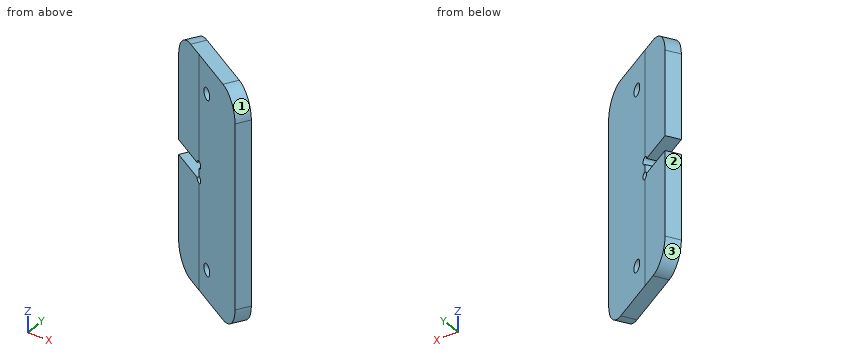
```python
from build123d import *

# Parameters (mm, degrees)
BOSS_EXTRUDE1_DEPTH      = 44.5
BOSS_EXTRUDE1_DEPTH_BACK = 50.5
SKETCH2_W                = 16.785504055
SKETCH2_H                = 44.5
BOSS_EXTRUDE2_DEPTH      = 6
FILLET1_R                = 10
SKETCH3_R                = 1.5
SKETCH3_R_2              = 2.4
CUT_EXTRUDE1_DEPTH       = 549.376643642


with BuildPart() as part:
    # Sketch1 → Boss-Extrude1 (new, two sides: drawn at the far end of the back side and taken through both)
    with BuildSketch(Plane.XY.offset(-25).offset(-BOSS_EXTRUDE1_DEPTH_BACK)):
        Polygon((724, 137.920851515), (698.573213095, 153.84185989), (701.75741477, 158.927217271), (727.184201675, 143.006208896), align=None)
    extrude(amount=BOSS_EXTRUDE1_DEPTH + BOSS_EXTRUDE1_DEPTH_BACK)

    # Sketch2 → Boss-Extrude2 (add)
    with BuildSketch(Plane(origin=(269.130391352, 429.817066188, 0), x_dir=(0.8475595635030609, -0.5307002791731893, 0), z_dir=(0.5307002791731893, 0.8475595635030609, 0))):
        with Locations((502.045737546, 53.25)):
            Rectangle(SKETCH2_W, SKETCH2_H)
        with Locations((502.045737546, 2.75)):
            Rectangle(SKETCH2_W, SKETCH2_H)
    extrude(amount=-BOSS_EXTRUDE2_DEPTH)

    # Fillet1
    fillet1_edges = [part.edges().sort_by_distance(p)[0] for p in [
        (725.592100838, 140.463530205, -75.5),
        (725.592100838, 140.463530205, 19.5),
        (685.938599442, 165.292610269, -75.5),
        (685.938599442, 165.292610269, 19.5),
    ]]
    fillet(fillet1_edges, radius=FILLET1_R)

    # Sketch3 → Cut-Extrude1 (cut, through all)
    with BuildSketch(Plane(origin=(269.130391352, 429.817066188, 0), x_dir=(0.8475595635030609, -0.5307002791731893, 0), z_dir=(0.5307002791731893, 0.8475595635030609, 0))):
        with Locations((510.438489573, 25)):
            Circle(SKETCH3_R)
        with Locations((510.438489573, 31)):
            Circle(SKETCH3_R)
        with Locations(Location((517.045737546, -7.5, 0), (0, 0, 180))):
            Circle(SKETCH3_R_2)
        with Locations(Location((517.045737546, 63.5, 0), (0, 0, 180))):
            Circle(SKETCH3_R_2)
    extrude(amount=-CUT_EXTRUDE1_DEPTH, mode=Mode.SUBTRACT)


solid = part.part
```
The model under review builds one solid part; all positions refer to its coordinate system, in mm. Face numbers are marked on the shaded views. Coordinates: 2 decimals unless noted, no trailing zeros. Write each loop counter-clockwise with the first axis right and the second up, starting at its lowest first coordinate (ties: lowest second). Pieces come first, ordered by that corner, then holes.
1) We need section B-B on z = -5.5. State the section outline as (x, y) points.
2) We need section A-A on z = -62.5. State the section outline as (x, y) points.
3) We need section C-C on x = 711. State the section outline as (y, z) points, then the cut area to 3 significant figures.
4) The part is to be moulded in two halves that separate along Z. For the marked faces 1, 2 and 3, say which applies: pulls with the +Z half, pulls with the -Z half, needs draft (parallel to the pull), parting line crosses it, or undercut.
5) Clearance check with flat-ended pins moving along their axes: pin 1 Ø1.5 at (y, z) = (150, 7.5) entering from -X; pin 2 Ø3 at (x, z) = (717, 4.5) entering from +Y; pin 3 Ø10 at (y, z) = (156.5, -22.5) entering from +X. State where each tip first meets the part, or that it passes through.
6) To check wall thickness, follow probe 1 along Z at (x, y) = (696, 160.75); probe 2 along Y at (x, z) = (707.5, -52); probe 3 along X at (y, z) = (166.75, 10.5). State the ranges of each line that lie inside material, in increasing order.
Answer list:
1. outline: (684.35, 162.75) - (724, 137.92) - (727.18, 143.01) - (687.53, 167.84) - close
2. outline: (684.35, 162.75) - (702.32, 151.49) - (705.51, 156.58) - (687.53, 167.84) - close; (706.02, 149.18) - (724, 137.92) - (727.18, 143.01) - (709.21, 154.26) - close
3. outline: (146.06, -75.5) - (153.14, -75.5) - (153.14, 19.5) - (146.06, 19.5) - close
3. area: 673 mm2
4. face 1: pulls with the +Z half
4. face 2: needs draft
4. face 3: pulls with the -Z half
5. pin 1: stops at x = 706.33
5. pin 2: stops at y = 150.32
5. pin 3: stops at x = 713.62
6. probe 1: z = -75.5 to -31, -25 to 19.5
6. probe 2: y = 148.25 to 155.33
6. probe 3: x = 686.91 to 689.26
